from build123d import *

# Parameters (mm, degrees)
F0_W     = 300
F0_H     = 400
F1_DEPTH = 19
F2_R     = 52.5
F3_DEPTH = 6
F5_DEPTH = 8
F6_W     = 30
F6_H     = 30
F7_DEPTH = 11


with BuildPart() as f1:
    # F0 (on Front) → F1 (new body)
    with BuildSketch(Plane.XZ):
        with Locations((-48.081684, 43.9321)):
            Rectangle(F0_W, F0_H)
    extrude(amount=F1_DEPTH)

    # F2 (on face) → F3 (cut)
    with BuildSketch(Plane.XZ.offset(19)):
        with Locations((-48.081684, -1.5679)):
            Circle(F2_R)
    extrude(amount=-F3_DEPTH, mode=Mode.SUBTRACT)

    # F4 (on face) → F5 (cut)
    with BuildSketch(Plane(origin=(0, 0, 0), x_dir=(-1, 0, 0), z_dir=(0, 1, 0))):
        Polygon((-91.418316, 233.9321), (-91.418316, -134.0679), (-61.418316, -134.0679), (-61.418316, 203.9321), (-49.918316, 203.9321), (-49.918316, -134.0679), (21.581684, -134.0679), (21.581684, 203.9321), (33.081684, 203.9321), (33.081684, -134.0679), (104.581684, -134.0679), (104.581684, 203.9321), (116.081684, 203.9321), (116.081684, -134.0679), (187.581684, -134.0679), (187.581684, 233.9321), (157.581684, 233.9321), (157.581684, -104.0679), (146.081684, -104.0679), (146.081684, 233.9321), (74.581684, 233.9321), (74.581684, -104.0679), (63.081684, -104.0679), (63.081684, 233.9321), (-8.418316, 233.9321), (-8.418316, -104.0679), (-19.918316, -104.0679), (-19.918316, 233.9321), align=None)
    extrude(amount=-F5_DEPTH, mode=Mode.SUBTRACT)

    # F6 (on face) → F7 (cut)
    with BuildSketch(Plane(origin=(0, -8, 0), x_dir=(-1, 0, 0), z_dir=(0, 1, 0))):
        with Locations((-76.418316, -119.0679)):
            Rectangle(F6_W, F6_H)
    extrude(amount=-F7_DEPTH, mode=Mode.SUBTRACT)


solid = f1.part
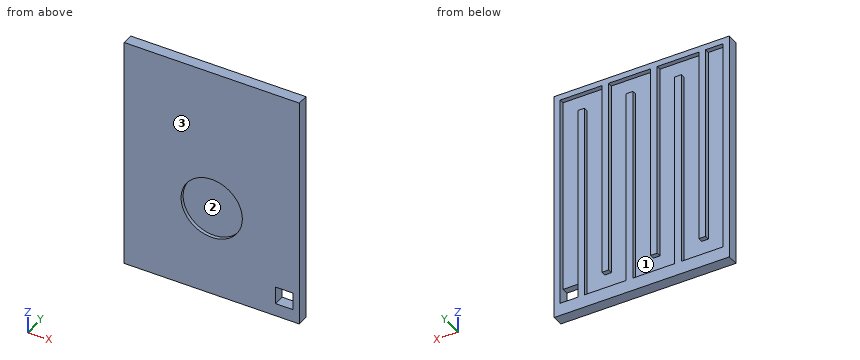
Read the model definition and answer for the solid it produces. Units are mm, in the model's axes. Face numbers are marked on the shaded views. Coordinates: 2 decimals unless noted, no trailing zeros. Loops run counter-clockwise (first coordinate to the right, second up) from the corner with the lowest first, then second, coordinate; pieces in that order, holes last. Notation, with made-up numbers: (83, -39.5) -> (109, -39.5) arc R13 ccw to (109, -29.5) -> close; hole circle Ø4 at (81, 30). An arc over 180 degrees is marked (long way). Answer in a Markdown table with one row per item.
Item 1: Straight lines are drawn through the part: line 1 along Z through (x, y) = (-30, -2); line 2 along Z through (x, y) = (48, -2.5); line 3 along X through (y, z) = (-17, -121). For each, find the intervals that lie inside material, in ascending order. Write a range as [from, to].
Returned:
| item | result |
|---|---|
| line 1 | z = [-156.07, 203.93], [233.93, 243.93] |
| line 2 | z = [-156.07, -134.07], [233.93, 243.93] |
| line 3 | x = [-198.08, 61.42], [91.42, 101.92] |
Item 2: A cutting plane is placed at D-D on x = -15.5. Determine the outline of the cut face in (y, z), plus the area to 3 significant figures.
Returned:
| item | result |
|---|---|
| outline | (-19, -156.07) -> (0, -156.07) -> (0, -134.07) -> (-8, -134.07) -> (-8, 233.93) -> (0, 233.93) -> (0, 243.93) -> (-19, 243.93) -> (-19, 39.6) -> (-13, 39.6) -> (-13, -42.73) -> (-19, -42.73) -> close |
| area | 4,160 mm^2 |
Item 3: For a pull along Z with two mould halves and no side action, classify the marked faces 1, 2 and 3 as released by +Z, released by -Z, zero draft, split by the parting line, or undercut.
Returned:
| item | result |
|---|---|
| face 1 | undercut |
| face 2 | undercut |
| face 3 | zero draft |
Item 4: This flat-tipped pin is pushed along its axis until it touches: P1, Ø6, axis at x = 2.5, z = 164, coming from the +Y side. Where does it stop, or does it pass through?
Returned:
| item | result |
|---|---|
| P1 | stops at y = -8 |
Item 5: A cutting plane is placed at B-B on x = -138.5. Determine the outline of the cut face in (y, z).
Returned:
| item | result |
|---|---|
| outline | (-19, -156.07) -> (0, -156.07) -> (0, -134.07) -> (-8, -134.07) -> (-8, 233.93) -> (0, 233.93) -> (0, 243.93) -> (-19, 243.93) -> close |
